Work out the finished part from the listing and answer in its coordinate system (mm). Round coordinates to 2 decimals unless told otherwise and drop trailing zeros. Loops run counter-clockwise (first coordinate to the right, second up) from the corner with the lowest first, then second, coordinate; pieces in that order, holes last. Notation, with made-up numbers: (63, 67) -> (100, 67) arc R18 cw to (100, 92) -> close; hole circle Ø5 at (80.25, 7). An arc over 180 degrees is marked (long way). Use one line per item in the form item = value.
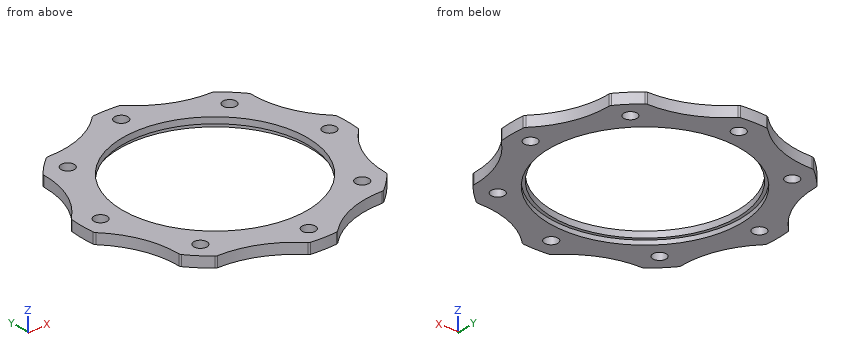
```python
from build123d import *

# Parameters (mm, degrees)
SKETCH_1_R               = 125
SKETCH_1_R_2             = 87
SKETCH_1_R_3             = 6.25
EXTRUDE_1_DEPTH          = 10
CUT_EXTRUDE_3_DEPTH      = 178.059312096
PATTERN_CIRCULAR_1_COUNT = 8
SKETCH_4_R               = 90
CUT_EXTRUDE_4_DEPTH      = 4.2


with BuildPart() as part:
    # Эскиз1 → Бобышка-Вытянуть1 (new body)
    with BuildSketch(Plane.XY):
        Circle(SKETCH_1_R)
        with Locations(Location((0, 0, 0), (0, 0, 180))):
            Circle(SKETCH_1_R_2, mode=Mode.SUBTRACT)
        with Locations((76.013978978, 76.013978978)):
            Circle(SKETCH_1_R_3, mode=Mode.SUBTRACT)
        with Locations((107.5, 0)):
            Circle(SKETCH_1_R_3, mode=Mode.SUBTRACT)
        with Locations((76.013978978, -76.013978978)):
            Circle(SKETCH_1_R_3, mode=Mode.SUBTRACT)
        with Locations((0, -107.5)):
            Circle(SKETCH_1_R_3, mode=Mode.SUBTRACT)
        with Locations((-76.013978978, -76.013978978)):
            Circle(SKETCH_1_R_3, mode=Mode.SUBTRACT)
        with Locations((-107.5, 0)):
            Circle(SKETCH_1_R_3, mode=Mode.SUBTRACT)
        with Locations((-76.013978978, 76.013978978)):
            Circle(SKETCH_1_R_3, mode=Mode.SUBTRACT)
        with Locations((0, 107.5)):
            Circle(SKETCH_1_R_3, mode=Mode.SUBTRACT)
    extrude(amount=EXTRUDE_1_DEPTH)

    # Эскиз3 → Вырез-Вытянуть3 (cut, symmetric)
    with BuildSketch(Plane.XY.offset(10)):
        with BuildLine():
            ThreePointArc((-12.208800164, 124.402352062), (-13.211334731, 124.122533958), (-14.057918159, 123.517000946))
            ThreePointArc((-14.057918159, 123.517000946), (-43.051886141, 103.936447408), (-77.399259701, 97.28015822))
            ThreePointArc((-77.399259701, 97.28015822), (-78.426061083, 97.109709837), (-79.332821353, 96.598672124))
            ThreePointArc((-79.332821353, 96.598672124), (-47.835429046, 115.484941564), (-12.208800164, 124.402352062))
        make_face()
    cut_extrude_3 = extrude(amount=CUT_EXTRUDE_3_DEPTH, both=True, mode=Mode.SUBTRACT)

    # Круговой массив1: Вырез-Вытянуть3 ×8 about axis
    pattern_circular_1_axis = Axis((0, 0, 0), (0, 0, -1))
    for i in range(1, PATTERN_CIRCULAR_1_COUNT):
        add(cut_extrude_3.rotate(pattern_circular_1_axis, i * 360 / PATTERN_CIRCULAR_1_COUNT), mode=Mode.SUBTRACT)

    # Эскиз4 → Вырез-Вытянуть4 (cut)
    with BuildSketch(Plane(origin=(0, 0, 0), x_dir=(-1, 0, 0), z_dir=(0, 0, -1))):
        Circle(SKETCH_4_R)
    extrude(amount=-CUT_EXTRUDE_4_DEPTH, mode=Mode.SUBTRACT)


solid = part.part
```
(1) Find section A-A, the plane x = 0. Write down the section's boundary in (y, z).
Completed:
outline = (-125, 0) -> (-113.75, 0) -> (-113.75, 10) -> (-125, 10) -> close; (-101.25, 0) -> (-90, 0) -> (-90, 4.2) -> (-87, 4.2) -> (-87, 10) -> (-101.25, 10) -> close; (87, 4.2) -> (90, 4.2) -> (90, 0) -> (101.25, 0) -> (101.25, 10) -> (87, 10) -> close; (113.75, 0) -> (125, 0) -> (125, 10) -> (113.75, 10) -> close
(2) Given P1, Ø10, axis at x = 76.01, y = 76.01, coming from the -Z side; P2, Ø3, axis at y = 21, z = 8.5, coming from the +X side; P3, Ø2, axis at x = 96, z = 3.5, coming from the -Y side; P4, Ø6, axis at x = 51, z = 4.5, coming from the +Y side, each flat-ended and moving along its own axis, determine where each tip first touches the part or whether it passes through.
Completed:
P1 = through
P2 = 118.42
P3 = -81.24
P4 = 102.06
(3) Find section D-D, the plane x = 107.5. Write down the section's boundary in (y, z).
Completed:
outline = (-35.49, 0) -> (-6.25, 0) -> (-6.25, 10) -> (-35.49, 10) -> close; (6.25, 0) -> (35.49, 0) -> (35.49, 10) -> (6.25, 10) -> close
(4) Find section C-C, the plane y = 48.5. Write down the section's boundary in (x, z), then the cut area to 3 significant figures.
Completed:
outline = (-101.89, 0) -> (-75.81, 0) -> (-75.81, 4.2) -> (-72.23, 4.2) -> (-72.23, 10) -> (-101.89, 10) -> close; (72.23, 4.2) -> (75.81, 4.2) -> (75.81, 0) -> (101.89, 0) -> (101.89, 10) -> (72.23, 10) -> close
area = 563 mm2
(5) Consider L1, parallel to Y at x = 0, z = 1.2; L2, parallel to Y at x = 0, z = 6; L3, parallel to X at y = -3.5, z = 9.75. Determine where each line is inside the solid, lowest interval first.
Completed:
L1 = -125 to -113.75, -101.25 to -90, 90 to 101.25, 113.75 to 125
L2 = -125 to -113.75, -101.25 to -87, 87 to 101.25, 113.75 to 125
L3 = -124.95 to -112.68, -102.32 to -86.93, 86.93 to 102.32, 112.68 to 124.95
